from build123d import *

# Parameters (mm, degrees)
BOSS_EXTRUDE1_DEPTH = 38.1
CHAMFER1_SIZE       = 11.43
CHAMFER1_SIZE2      = 19.797340731


with BuildPart() as part:
    # Sketch1 → Boss-Extrude1 (new body)
    with BuildSketch(Plane.XY):
        with BuildLine():
            Line((0, 0), (50.8, 0))
            Line((50.8, 0), (50.8, 25.4))
            Line((50.8, 25.4), (0, 25.4))
            ThreePointArc((0, 25.4), (12.7, 12.7), (0, 0))
        make_face()
    extrude(amount=BOSS_EXTRUDE1_DEPTH)

    # Chamfer1
    chamfer1_edges = [part.edges().sort_by_distance(p)[0] for p in [
        (50.8, 0, 19.05),
    ]]
    chamfer1_side = [part.faces().sort_by_distance(p)[0] for p in [
        (25.4, 0, 19.05),
    ]]
    chamfer(chamfer1_edges, length=CHAMFER1_SIZE, length2=CHAMFER1_SIZE2, reference=chamfer1_side[0])


solid = part.part
Can you work these out from the model? Positions are in its coordinate system, mm. Give positions to 0.01 mm unless a question says otherwise; leave off trailing zeros. Order: outer loops, then holes, each group sorted by start corner. A loop starts at its lowest first (then second) coordinate and runs counter-clockwise, first axis right, second up. Notation, with made-up numbers: M 87.25,59 L 121.25,59 A20 cw 121.25,95 Z; hole C -14.5,-30 d10. An arc over 180 degrees is marked long. Use one line per item in the form item = value.
Item 1: Thinking about a two-plate mould opening in Y: for faces 1 (the cylindrical face through (12.697, 12.979, 18.783)), 2 (the flat face through (45.165, 10.037, 18.783)), 3 (the flat face through (50.8, 23, 19)), which applies, pulls with the +Y half, pulls with the -Y half, needs draft (parallel to the pull), parting line crosses it, or undercut?
Values follow:
face_1 = undercut
face_2 = pulls with the -Y half
face_3 = needs draft
Item 2: If we section it at C-C, the plane y = 12.5: Write out the boundary of the cut face in (x, z).
Values follow:
outline = M 12.7,0 L 46.59,0 L 46.59,38.1 L 12.7,38.1 Z
Item 3: If we section it at B-B, the plane z = 18: Write out the boundary of the cut face in (x, y), and give its area (3 significant figures).
Values follow:
outline = M 0,0 L 39.37,0 L 50.8,19.8 L 50.8,25.4 L 0,25.4 A12.7 cw Z
area = 924 mm^2
Item 4: Will these pins go through, and if not, where does the flat tip stop? pin 1 Ø1.5 at (y, z) = (3.5, 5) entering from -X; pin 2 Ø3 at (x, y) = (21.5, 22) entering from -Z; pin 3 Ø5 at (y, z) = (8, 25.5) entering from -X; pin 4 Ø8 at (y, z) = (5.5, 4) entering from -X.
Values follow:
pin_1 = 7.89
pin_2 = 0
pin_3 = 10.46
pin_4 = 5.99
Item 5: If we section it at A-A, the plane x = 6: Write out the boundary of the cut face in (y, z), and give its area (3 significant figures).
Values follow:
outline = M 0,0 L 1.51,0 L 1.51,38.1 L 0,38.1 Z; M 23.89,0 L 25.4,0 L 25.4,38.1 L 23.89,38.1 Z
area = 115 mm^2
Item 6: If I drill on line 1 along X through (y, z) = (19.25, 7); line 2 along X through (y, z) = (11.5, 29); line 3 along Y through (x, z) = (40, 13), over which ranges is the centre line in solid material (lowest first)? Write a range as [from, to].
Values follow:
line_1 = [10.88, 50.48]
line_2 = [12.64, 46.01]
line_3 = [1.09, 25.4]
Item 7: If we section it at D-D, the plane x = 40: Write out the boundary of the cut face in (y, z).
Values follow:
outline = M 1.09,0 L 25.4,0 L 25.4,38.1 L 1.09,38.1 Z
